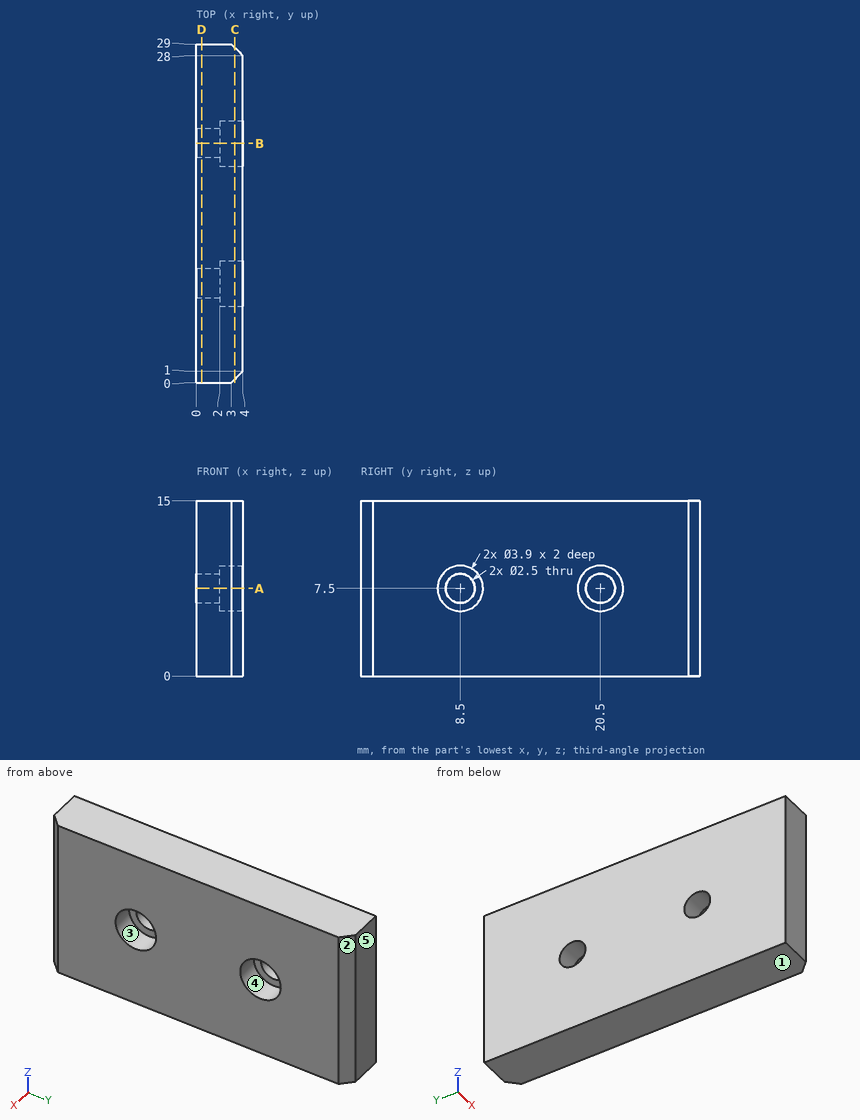
Design review of the part shown in the three views and the two pictorial views. Dimensions are in mm from the part's minimum x, y and z. A direction names the side the tool comes from. Give positions to 0.01 mm unless a question says otherwise; leave off trailing zeros. Loops run counter-clockwise (first coordinate to the right, second up) from the corner with the lowest first, then second, coordinate; pieces in that order, holes last. Notation, with made-up numbers: M -11.5,32.5 L 28.5,32.5 A21 ccw 28.5,55.5 Z; hole C 14,-14.75 d5. An arc over 180 degrees is marked long. Write item = value, one per line.
Q1. We need section D-D (x = 0.45). Give the boundary of the cut face in (y, z), plus the area to 3 significant figures.
Output values:
outline = M 0,0 L 29,0 L 29,15 L 0,15 Z; hole C 8.5,7.5 d2.5; hole C 20.5,7.5 d2.5
area = 425 mm^2
Q2. We need section C-C (x = 3.3). Give the boundary of the cut face in (y, z), plus the area to 3 significant figures.
Output values:
outline = M 0.3,0 L 28.7,0 L 28.7,15 L 0.3,15 Z; hole C 8.5,7.5 d3.9; hole C 20.5,7.5 d3.9
area = 402 mm^2
Q3. We need section B-B (y = 20.5). Give the boundary of the cut face in (x, z), plus the area to 3 significant figures.
Output values:
outline = M 0,0 L 4,0 L 4,5.55 L 2,5.55 L 2,6.25 L 0,6.25 Z; M 0,8.75 L 2,8.75 L 2,9.45 L 4,9.45 L 4,15 L 0,15 Z
area = 47.2 mm^2
Q4. To check wall thickness, follow line 1 (Y direction, x = 2.6, z = 7.5); line 2 (Z direction, x = 1.1, y = 8.5); line 3 (Z direction, x = 3.8, y = 19.5). State the ranges of each line that lie inside material, in increasing order. Write a range as [from, to].
Output values:
line_1 = [0, 6.55], [10.45, 18.55], [22.45, 29]
line_2 = [0, 6.25], [8.75, 15]
line_3 = [0, 5.83], [9.17, 15]
Q5. For the marked faces 4 and 5, list the 3-axis set-ups (+Z, -Z, +X, -X, +Y, -Y) from which the entire face can be reached by the end or side of a thin tool; tool diameter is ignored.
Output values:
face_4 = +X
face_5 = +Z, -Z, +X, -X, +Y
Q6. Insertion check: pin 1 (4.5 mm diameter, centred on y = 20.5, z = 7.5, fed in from +X). The pin has a flat end and moves straight along its axis. Give the tip position at first contact, or say it passes through.
Output values:
pin_1 = 4
Q7. We need section A-A (z = 7.5). Give the boundary of the cut face in (x, y).
Output values:
outline = M 0,0 L 3,0 L 4,1 L 4,6.55 L 2,6.55 L 2,7.25 L 0,7.25 Z; M 0,9.75 L 2,9.75 L 2,10.45 L 4,10.45 L 4,18.55 L 2,18.55 L 2,19.25 L 0,19.25 Z; M 0,21.75 L 2,21.75 L 2,22.45 L 4,22.45 L 4,28 L 3,29 L 0,29 Z
Q8. Draft analysis for pull direction Z (two halves, no side actions). For the marked faces 1, 2 and 3, state which applies: +Z half, -Z half, draft (parallel to the pull), parting line (faces both ways), or undercut.
Output values:
face_1 = -Z half
face_2 = draft
face_3 = undercut
